```python
from build123d import *

# Parameters (mm, degrees)
F7_R          = 7
F7_R_2        = 4
F8_DEPTH      = 25
F9_DEPTH      = 1
F7_R_3        = 8
F10_DEPTH     = 1
F11_DEPTH     = 3
F13_DEPTH     = 16
F14_R         = 2.9021632183
F15_DEPTH     = 12.5
F16_T4_DEPTH  = 21.5714554244
F16_S5_R      = 8
F16_T6_DEPTH  = 12
F16_T10_DEPTH = 21.5714554244
F16_S11_R     = 8
F16_T12_DEPTH = 12
F16_T16_ANGLE = 175.2944368931
F16_T18_ANGLE = 175.2944368931


# Not quite as in the source:
# - a fillet or chamfer that OpenCascade refuses, or shapes differently, is made with other operations: its cross-section is extruded or revolved along the edge and cut away or added


with BuildPart() as f8:
    # F7 (on Top) → F8 (new body)
    with BuildSketch(Plane.XY):
        Circle(F7_R)
        Circle(F7_R_2, mode=Mode.SUBTRACT)
    extrude(amount=F8_DEPTH)

    # F7 (on Top) → F9 (join)
    with BuildSketch(Plane.XY):
        Circle(F7_R_2)
    extrude(amount=F9_DEPTH)

    # F7 (on Top) → F10 (join)
    with BuildSketch(Plane.XY):
        Circle(F7_R_3)
        Circle(F7_R, mode=Mode.SUBTRACT)
    extrude(amount=F10_DEPTH)

    # F7 (on Top) → F11 (join)
    with BuildSketch(Plane.XY):
        Circle(F7_R_3)
        Circle(F7_R, mode=Mode.SUBTRACT)
        Circle(F7_R)
        Circle(F7_R_2, mode=Mode.SUBTRACT)
        Circle(F7_R_2)
    extrude(amount=-F11_DEPTH)

    # F12 (on face) → F13 (join)
    with BuildSketch(Plane(origin=(0, 0, -3), x_dir=(1, 0, 0), z_dir=(0, 0, -1))):
        with BuildLine():
            Line((-4, -6.9282032303), (-4, 6.9282032303))
            ThreePointArc((-4, 6.9282032303), (-8, 0), (-4, -6.9282032303))
        make_face()
        with BuildLine():
            ThreePointArc((8, 0), (6.9282032303, 4), (4, 6.9282032303))
            Line((4, 6.9282032303), (4, -6.9282032303))
            ThreePointArc((4, -6.9282032303), (6.9282032303, -4), (8, 0))
        make_face()
    extrude(amount=F13_DEPTH)

    # F14 (on Right) → F15 (cut, symmetric)
    with BuildSketch(Plane.YZ):
        with Locations((0, -12.0717967697)):
            Circle(F14_R)
    extrude(amount=F15_DEPTH, both=True, mode=Mode.SUBTRACT)

    # F16: chamfer of 1.5 on 5 edges, made by hand


with BuildPart() as f16_tool2:
    # F16_s3 → F16_t4 (new body)
    with BuildSketch(Plane.XZ.offset(10.7857277122)):
        Polygon((2.5, -3), (4, -4.5), (4, -3), align=None)
    extrude(amount=-F16_T4_DEPTH)

    # F16_s5 → F16_t6 (intersect, symmetric)
    with BuildSketch(Plane.XY.offset(-3.8)):
        Circle(F16_S5_R)
    extrude(amount=F16_T6_DEPTH, both=True, mode=Mode.INTERSECT)


with BuildPart() as f8_1:
    add(f8.part)

    # F16_t1: union F16_tool2
    add(f16_tool2.part)


with BuildPart() as f16_tool8:
    # F16_s9 → F16_t10 (new body)
    with BuildSketch(Plane.XZ.offset(-10.7857277122)):
        Polygon((-2.5, -3), (-4, -4.5), (-4, -3), align=None)
    extrude(amount=F16_T10_DEPTH)

    # F16_s11 → F16_t12 (intersect, symmetric)
    with BuildSketch(Plane.XY.offset(-3.8)):
        Circle(F16_S11_R)
    extrude(amount=F16_T12_DEPTH, both=True, mode=Mode.INTERSECT)


with BuildPart() as f8_2:
    add(f8_1.part)

    # F16_t7: union F16_tool8
    add(f16_tool8.part)

    # F16_s13 → F16_t14 (revolve, cut)
    with BuildSketch(Plane.XZ):
        Polygon((7, 23.5), (5.5, 25), (7, 25), align=None)
    revolve(axis=Axis((0, 0, 25), (0, 0, 1)), mode=Mode.SUBTRACT)

    # F16_s15 → F16_t16 (revolve, cut)
    with BuildSketch(Plane(origin=(0, 0, 0), x_dir=(0, 0, 1), z_dir=(-0.9991570013, 0.0410522451, 0))):
        Polygon((-17.5, 8), (-19, 6.5), (-19, 8), align=None)
    revolve(axis=Axis((0, 0, -19), (0, 0, -1)), revolution_arc=F16_T16_ANGLE, mode=Mode.SUBTRACT)

    # F16_s17 → F16_t18 (revolve, cut)
    with BuildSketch(Plane(origin=(0, 0, 0), x_dir=(0, 0, 1), z_dir=(0.9991570013, -0.0410522451, 0))):
        Polygon((-17.5, 8), (-19, 6.5), (-19, 8), align=None)
    revolve(axis=Axis((0, 0, -19), (0, 0, -1)), revolution_arc=F16_T18_ANGLE, mode=Mode.SUBTRACT)


solid = f8_2.part
```
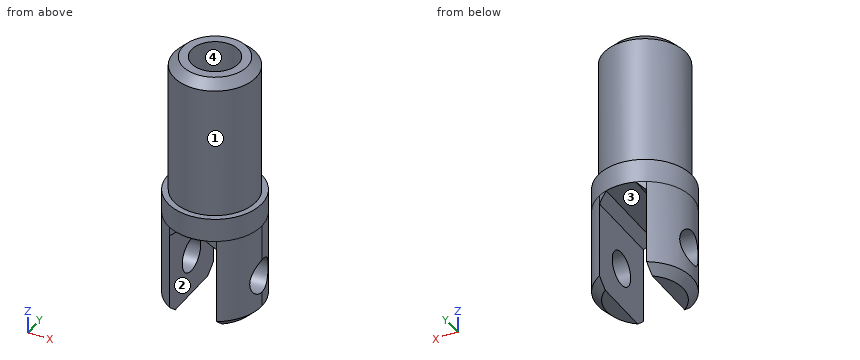
Source: CAD feature listing. Evaluate the final solid. Frame: model axes, mm. Face numbers are marked on the shaded views. A direction names the side the tool comes from. Give positions to 0.01 mm unless a question says otherwise; leave off trailing zeros. Loops run counter-clockwise (first coordinate to the right, second up) from the corner with the lowest first, then second, coordinate; pieces in that order, holes last. Notation, with made-up numbers: (17, 20.25) -> (32, 20.25) arc R30 ccw to (32, 46.25) -> close; hole circle Ø8 at (75, 36.5). An arc over 180 degrees is marked (long way). Use a Markdown table: item, result. Add a question column.
(1) Section query A-A (z = -5). Output: boundary loops of the cut face in (x, y), then the cut area to 3 significant figures.
(2) Ray query, line 1 (Y direction, x = 0, z = 7.5); line 2 (X direction, y = -0.25, z = 10); line 3 (Z direction, x = -2.25, y = -4). Return the intervals inside material, ascending.
(3) Section query B-B (z = 5). Output: boundary loops of the cut face in (x, y).
(4) First-contact query: pin 1 Ø8 at (y, z) = (4, 5.5) entering from -X; pin 2 Ø1 at (x, y) = (0, 2.5) entering from +Z; pin 3 Ø5.5 at (x, y) = (-1, 3.5) entering from -Z. Flat tips, straight axial feed; report the tip coordinate or a pass-through.
(5) Section query D-D (y = 1.75). Count the separate pieces of the cut face and the enclosed holes in it, then the cut area to 3 significant figures.
(6) Section query C-C (x = 0). Output: boundary loops of the cut face in (y, z).
(7) Access query for the marked faces 3 and 4. Directions: +Z, -Z, +X, -X, +Y, -Y. A direction counts if a zero-diameter tool reaches every point of the face in a straight line with its end or side. Return the directions, or none.
(8) Pull-direction query (X, two-part tool) for the marked faces 1 and 2; classes: +X half, -X half, draft (parallel to the pull), parting line (faces both ways), or undercut.
Checked values:
| question | item | result |
|---|---|---|
| 1 | outline | (-4, -6.93) -> (-4, 6.93) arc R8 ccw to start; (4, -6.93) arc R8 ccw to (4, 6.93) -> close |
| 1 | area | 78.6 mm^2 |
| 2 | line 1 | -7 to -4, 4 to 7 |
| 2 | line 2 | -7 to -3.99, 3.99 to 7 |
| 2 | line 3 | -3 to 25 |
| 3 | outline | circle Ø14 at (0, 0); hole circle Ø8 at (0, 0) |
| 4 | pin 1 | x = -7 |
| 4 | pin 2 | z = 1 |
| 4 | pin 3 | z = -4.25 |
| 5 | separate pieces | 3 |
| 5 | enclosed holes | 0 |
| 5 | area | 299 mm^2 |
| 6 | outline | (-8, -3) -> (8, -3) -> (8, 1) -> (7, 1) -> (7, 23.5) -> (5.5, 25) -> (4, 25) -> (4, 1) -> (-4, 1) -> (-4, 25) -> (-5.5, 25) -> (-7, 23.5) -> (-7, 1) -> (-8, 1) -> close |
| 7 | face 3 | -Z, +Y, -Y |
| 7 | face 4 | +Z |
| 8 | face 1 | parting line |
| 8 | face 2 | undercut |
